```python
from build123d import *

# Parameters (mm, degrees)
CROQUIS1_W              = 120
CROQUIS1_H              = 140
SALIENTE_EXTRUIR1_DEPTH = 5
CROQUIS2_R              = 2
CROQUIS2_R_2            = 1.5
CORTAR_EXTRUIR1_DEPTH   = 5
CROQUIS3_W              = 4
CROQUIS3_H              = 110.000000561
CORTAR_EXTRUIR2_DEPTH   = 5
CROQUIS5_R              = 30
CORTAR_EXTRUIR3_DEPTH   = 5
REDONDEO2_R             = 10
REDONDEO3_R             = 60


with BuildPart() as part:
    # Croquis1 → Saliente-Extruir1 (new body)
    with BuildSketch(Plane.XY):
        Rectangle(CROQUIS1_W, CROQUIS1_H)
    extrude(amount=SALIENTE_EXTRUIR1_DEPTH)

    # Croquis2 → Cortar-Extruir1 (cut)
    with BuildSketch(Plane.XY.offset(5)):
        with Locations((-40, 30)):
            Circle(CROQUIS2_R)
        with Locations((40, 30)):
            Circle(CROQUIS2_R)
        with Locations((0, 65)):
            Circle(CROQUIS2_R)
        with Locations((0, -45)):
            Circle(CROQUIS2_R)
        with Locations((-20, 60.5)):
            Circle(CROQUIS2_R_2)
        with Locations((20, 60.5)):
            Circle(CROQUIS2_R_2)
        with Locations((20, 20.5)):
            Circle(CROQUIS2_R_2)
    extrude(amount=-CORTAR_EXTRUIR1_DEPTH, mode=Mode.SUBTRACT)

    # Croquis3 → Cortar-Extruir2 (cut)
    with BuildSketch(Plane.XY.offset(5)):
        with Locations((0, 9.999999746)):
            Rectangle(CROQUIS3_W, CROQUIS3_H)
    extrude(amount=-CORTAR_EXTRUIR2_DEPTH, mode=Mode.SUBTRACT)

    # Croquis5 → Cortar-Extruir3 (cut)
    with BuildSketch(Plane.XY.offset(5)):
        with Locations((-60, 70)):
            Circle(CROQUIS5_R)
        with Locations((60, 70)):
            Circle(CROQUIS5_R)
    extrude(amount=-CORTAR_EXTRUIR3_DEPTH, mode=Mode.SUBTRACT)

    # Redondeo2
    redondeo2_edges = [part.edges().sort_by_distance(p)[0] for p in [
        (-30, 70, 2.5),
        (-60, 40, 2.5),
        (60, 40, 2.5),
        (30, 70, 2.5),
    ]]
    fillet(redondeo2_edges, radius=REDONDEO2_R)

    # Redondeo3
    redondeo3_edges = [part.edges().sort_by_distance(p)[0] for p in [
        (60, -70, 2.5),
        (-60, -70, 2.5),
    ]]
    fillet(redondeo3_edges, radius=REDONDEO3_R - 0.0001)  # a hair under: the kernel refuses the full size


solid = part.part
```
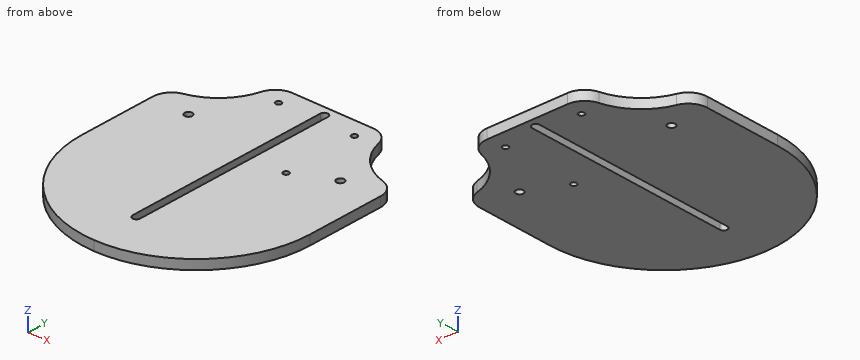
Input: part model. Units: mm. Frame: model coordinates. Give positions to 0.01 mm unless a question says otherwise; leave off trailing zeros. Order: outer loops, then holes, each group sorted by start corner. A loop starts at its lowest first (then second) coordinate and runs counter-clockwise, first axis right, second up. Notation, with made-up numbers: M 23,63 L 63,63 A27 ccw 63,83 Z; hole C 43,80.25 d4. An arc over 180 degrees is marked long. One line per question, with ' | ' between items.
1) Section C-C on y = 60.5. Output: boundary loops of the cut face in (x, z).
Filled in:
outline: M -31.54,0 L -21.5,0 L -21.5,5 L -31.54,5 Z; M -18.5,0 L -2,0 L -2,5 L -18.5,5 Z; M 2,0 L 18.5,0 L 18.5,5 L 2,5 Z; M 21.5,0 L 31.54,0 L 31.54,5 L 21.5,5 Z
2) Section B-B on z = 1.3. State how many separate pieces and enclosed holes the cut face has, and give its area (3 significant figures).
Filled in:
separate pieces: 1 | enclosed holes: 6 | area: 13,300 mm2
3) Section D-D on x = 40. Output: boundary loops of the cut face in (y, z), and give its area (3 significant figures).
Filled in:
outline: M -54.72,0 L 28,0 L 28,5 L -54.72,5 Z; M 32,0 L 47.64,0 L 47.64,5 L 32,5 Z | area: 492 mm2
4) Contact query for flat-ended pins moving along their axis: P1, Ø2.5, axis at x = -20, y = 60.5, coming from the +Z side; P2, Ø3, axis at x = -7, z = 2, coming from the -Y side. Output: stop coordinate, or through.
Filled in:
P1: passes through | P2: stops at y = -69.75
5) Ray query, L1, parallel to X at y = -10.5, z = 2.9; L2, parallel to X at y = 30.5, z = 4.2; L3, parallel to Y at x = 20, z = 2.95. Return the intervals inside material, ascending.
Filled in:
L1: x = -60 to -2, 2 to 60 | L2: x = -60 to -41.94, -38.06 to -2, 2 to 38.06, 41.94 to 60 | L3: y = -66.57 to 19, 22 to 59, 62 to 70
6) Section A-A on y = 14. Output: boundary loops of the cut face in (x, z).
Filled in:
outline: M -60,0 L -2,0 L -2,5 L -60,5 Z; M 2,0 L 60,0 L 60,5 L 2,5 Z
